Build history of the part. All positions in model axes, mm. A direction names the side the tool comes from. Give positions to 0.01 mm unless a question says otherwise; leave off trailing zeros. Order: outer loops, then holes, each group sorted by start corner. A loop starts at its lowest first (then second) coordinate and runs counter-clockwise, first axis right, second up. Notation, with made-up numbers: (-34.75, 39.5) - (-25.75, 39.5) arc R32 ccw to (-25.75, 73.5) - close; hole circle Ø7 at (45.25, -13.75). An arc over 180 degrees is marked (long way). Answer in a Markdown table with one row per item.
Autodesk Inventor part; units mm, degrees
ref_plane "YZ Plane" through (0, 0, 0) normal (1, 0, 0) x (0, 1, 0)
ref_plane "XZ Plane" through (0, 0, 0) normal (0, 1, 0) x (-1, 0, 0)
ref_plane "XY Plane" through (0, 0, 0) normal (0, 0, 1) x (1, 0, 0)
sketch "スケッチ1" plane through (0, 0, 0) normal (1, 0, 0) x (0, 1, 0)
  circle A0 centre (0, 0) radius 10
  circle A1 centre (0, -10) radius 1.35
  circle A2 centre (8.6603, 5) radius 1.35
  circle A3 centre (-8.6603, 5) radius 1.35
  circle A4 centre (0, 0) radius 5
  line L0 (0, 0) -> (0, 50)
  circle A5 centre (0, 50) radius 22.5
  circle A6 centre (0, 0) radius 14
  line L1 (-14, 0) -> (-22.5, 50)
  line L2 (14, 0) -> (22.5, 50)
  line L3 (0, -14) -> (-11.62, -14)
  line L4 (-11.62, -14) -> (-14, 0)
  line L5 (0, -14) -> (11.62, -14)
  line L6 (11.62, -14) -> (14, 0)
  line L7 (0, 20) -> (-17.4, 20)
  line L8 (0, 20) -> (17.4, 20)
  dimension "d0" = 20
  dimension "d1" = 2.7
  dimension "d4" = 360
  dimension "d6" = 10
  dimension "d7" = 50
  dimension "d8" = 45
  dimension "d9" = 28
extrude "押し出し1" add sketch "スケッチ1" along normal blind 4 contours A0 A1 A3 A2 | A6 L6 L4 | A6 L1 L7 L0 | L0 L8 L2 A6 | L6 L5 A6 | A6 L3 L4
sketch "スケッチ2" plane through (0, -17.4, 20) normal (0, 0, 1) x (1, 0, 0)
  line L0 (0, 17.4) -> (30, 17.4)
  circle A0 centre (30, 17.4) radius 22.5
  circle A1 centre (30, 17.4) radius 18.5
  circle A2 centre (30, 17.4) radius 14
  circle A3 centre (48.5, 17.4) radius 1.35
  circle A4 centre (20.75, 33.4215) radius 1.35
  circle A5 centre (20.75, 1.3785) radius 1.35
  line L1 (0, 29.02) -> (0, 34.8)
  line L2 (0, 0) -> (0, 5.78)
  line L3 (0, 34.8) -> (0, 0)
  line L4 (4, 29.02) -> (4, 34.8)
  line L5 (4, 34.8) -> (7, 34.8)
  line L6 (7, 34.8) -> (30, 39.9)
  line L7 (4, 0) -> (4, 5.78)
  line L8 (4, 0) -> (7, 0)
  line L9 (7, 0) -> (30, -5.1)
  line L10 (4, 0) -> (0, 0)
  line L11 (0, 34.8) -> (4, 34.8)
  line L12 (0, 0) -> (0, 34.8)
  line L13 (0, 34.8) -> (4, 34.8)
  dimension "d14" = 37
  dimension "d12" = 30
  dimension "d13" = 45
  dimension "d15" = 28
  dimension "d16" = 2.7
  dimension "d19" = 360
  dimension "d21" = 3
  dimension "d22" = 3
extrude "押し出し2" add sketch "スケッチ2" along normal blind 2.5 contours L3 L1 L11 L5 L6 A0 L0 | L0 A0 L9 L8 L10 L2 L3 | A1 A4 A3 A5 | A0 L6 L9
fillet "フィレット1" radius 3 2 edges at (4, 0, 20) (0, 0, 22.5)
fillet "フィレット2" radius 3 2 edges at (2, -11.62, -14) (2, 11.62, -14)
sketch "スケッチ7" plane through (0, -17.4, 22.5) normal (0, 0, 1) x (1, 0, 0)
  circle A0 centre (30, 17.4) radius 14
  line L0 (30, 17.4) -> (182.95, 17.4)
  line L1 (30, 17.4) -> (182.95, 17.4) construction
  circle A1 centre (182.95, 17.4) radius 3.5
  circle A2 centre (182.95, 17.4) radius 10
  line L2 (182.95, 27.4) -> (50.1556, 27.4)
  arc A3 (30, -5.1) -> (30, 39.9) centre (30, 17.4) ccw
  line L3 (182.95, 27.4) -> (315.7444, 27.4) construction
  line L4 (182.95, 7.4) -> (50.1556, 7.4)
  point P0 (0, 17.4)
  dimension "d55" = 152.95
  dimension "d56" = 0
  dimension "d57" = 7
  dimension "d58" = 20
  dimension "d59" = 180
extrude "押し出し7" add sketch "スケッチ7" against normal blind 2.5 contours A3 L2 A2 L0 | L0 A2 L4 A3 | A2
fillet "フィレット3" radius 2 2 edges at (50.1556, 10, 21.25) (50.1556, -10, 21.25)
sketch "スケッチ9" plane through (0, -17.4, 22.5) normal (0, 0, 1) x (1, 0, 0)
  circle A0 centre (182.95, 17.4) radius 3.5
  circle A1 centre (182.95, 17.4) radius 3.5
  circle A2 centre (182.95, 17.4) radius 2
  point P0 (0, 17.4)
  dimension "d68" = 4
extrude "押し出し9" add sketch "スケッチ9" against normal blind 0.5
sketch "スケッチ10" plane through (0, -17.4, 20) normal (0, 0, -1) x (-1, 0, 0)
  circle A0 centre (-182.95, 17.4) radius 3.5
  circle A1 centre (-182.95, 17.4) radius 3.6
  point P0 (0, 17.4)
  dimension "d71" = 7.2
extrude "押し出し10" cut sketch "スケッチ10" against normal blind 2 contours A0 | A1
properties part number "motor_holder_2" material "アルミニウム 6061"
1. Drop flat-ended pins along their axis: P1, Ø15.5, axis at y = -5.5, z = 0, coming from the +X side; P2, Ø13.5, axis at x = 78.5, y = -7, coming from the -Z side; P3, Ø2, axis at x = 4.5, z = 21.5, coming from the +Y side. Give the stop position or say it passes through.
Check result:
| item | result |
|---|---|
| P1 | stops at x = 4 |
| P2 | stops at z = 20 |
| P3 | stops at y = 17.4 |
2. Cut at A-A on x = 145.5. Write the cut outline in (y, z).
Check result:
| item | result |
|---|---|
| outline | (-10, 20) - (10, 20) - (10, 22.5) - (-10, 22.5) - close |
3. Which spindle directions (+Z, -Z, +X, -X, +Y, -Y) get a long thin tool onto all of the face, cutting with end or side? Do faces 1 (the face through (41.22, 19.503, 21.232)), 2 (the face through (4, -0.2, 5.2)), 3 (the face through (186.547, 0.158, 20.986)). Say none if no direction does.
Check result:
| item | result |
|---|---|
| face 1 | +Z, -Z, +X, +Y |
| face 2 | -Z, +X, +Y, -Y |
| face 3 | -Z |
4. Two-plate mould, pull along X, no slides. Class faces 4 (the face through (184, -2, 22)), 5 (the face through (97, 0, 22.5)), 6 (the face through (18.339, 19.914, 21.232)), 7 (the face through (184.797, -0.766, 22.254)): +X half, -X half, draft (parallel to the pull), parting line (faces both ways), or undercut.
Check result:
| item | result |
|---|---|
| face 4 | undercut |
| face 5 | draft |
| face 6 | -X half |
| face 7 | undercut |
5. Probe line 1 (Y direction, x = 1, z = 0); line 2 (X direction, y = -15, z = 13); line 3 (Z direction, x = 157.5, y = 0.5). List the from-to ranges inside material, lowest first.
Check result:
| item | result |
|---|---|
| line 1 | y = -14 to -5, 5 to 14 |
| line 2 | x = 0 to 4 |
| line 3 | z = 20 to 22.5 |
